Can you work these out from the model? Positions are in its coordinate system, mm. Give positions to 0.01 mm unless a question says otherwise; leave off trailing zeros. Loops run counter-clockwise (first coordinate to the right, second up) from the corner with the lowest first, then second, coordinate; pieces in that order, holes last. Notation, with made-up numbers: (0.25, 19) -> (58.25, 19) arc R33 cw to (58.25, 53) -> close; hole circle Ø11 at (-23.75, -39). An arc over 180 degrees is marked (long way). Return JSON: item names as keys, results as strings. Group by question number.
Q1. I need wall thicknesses on line 1 along Z through (x, y) = (-13, 17.5); line 2 along Y through (x, z) = (27, 0.2); line 3 along X through (y, z) = (-4, 1). Which ranges of each line are inside material? Lowest first, please. Write a range as [from, to].
Q2. Suppose I cut it at A-A, the plane x = 21.5. Please give me the cut outline in (y, z).
Q3. Will this pin go through, and if not, where does the flat tip stop? pin 1 (0.8 mm diameter, centred on y = -9.5, z = 0.5, fed in from -X).
Q4. Suppose I cut it at B-B, the plane y = 16. Please give me the cut outline in (x, z), and give its area (3 significant figures).
```python
from build123d import *

# Parameters (mm, degrees)
F2_W     = 21.7
F2_H     = 24
F3_DEPTH = 2
F4_DEPTH = 1.5
F5_W     = 21.7
F5_H     = 24
F6_DEPTH = 2


with BuildPart() as f3:
    # F2 (on Top) → F3 (new body)
    with BuildSketch(Plane.XY):
        Polygon((32.5, 26.99), (-32.5, 26.99), (-32.5, 24.9966666667), (-10.8, 24.9966666667), (-10.8, 0.9966666667), (-32.5, 0.9966666667), (-32.5, -0.9966666667), (-10.8, -0.9966666667), (-10.8, -24.9966666667), (-32.5, -24.9966666667), (-32.5, -26.99), (32.5, -26.99), (32.5, -24.9966666667), (10.8, -24.9966666667), (10.8, -0.9966666667), (32.5, -0.9966666667), (32.5, 0.9966666667), (10.8, 0.9966666667), (10.8, 24.9966666667), (32.5, 24.9966666667), align=None)
        with Locations((21.65, 12.9966666667)):
            Rectangle(F2_W, F2_H)
        with Locations((-21.65, -12.9966666667)):
            Rectangle(F2_W, F2_H)
        with Locations((-21.65, 12.9966666667)):
            Rectangle(F2_W, F2_H)
        with Locations((21.65, -12.9966666667)):
            Rectangle(F2_W, F2_H)
    extrude(amount=-F3_DEPTH)

    # F2 (on Top) → F4 (join)
    with BuildSketch(Plane.XY):
        Polygon((32.5, 26.99), (-32.5, 26.99), (-32.5, 24.9966666667), (-10.8, 24.9966666667), (-10.8, 0.9966666667), (-32.5, 0.9966666667), (-32.5, -0.9966666667), (-10.8, -0.9966666667), (-10.8, -24.9966666667), (-32.5, -24.9966666667), (-32.5, -26.99), (32.5, -26.99), (32.5, -24.9966666667), (10.8, -24.9966666667), (10.8, -0.9966666667), (32.5, -0.9966666667), (32.5, 0.9966666667), (10.8, 0.9966666667), (10.8, 24.9966666667), (32.5, 24.9966666667), align=None)
    extrude(amount=F4_DEPTH)

    # F5 (on face) → F6 (join)
    with BuildSketch(Plane.XY.offset(1.5)):
        Polygon((10.8, -24.9966666667), (10.8, -0.9966666667), (32.5, -0.9966666667), (32.5, 0.9966666667), (10.8, 0.9966666667), (10.8, 24.9966666667), (32.5, 24.9966666667), (32.5, 26.99), (-32.5, 26.99), (-32.5, 24.9966666667), (-10.8, 24.9966666667), (-10.8, 0.9966666667), (-32.5, 0.9966666667), (-32.5, -0.9966666667), (-10.8, -0.9966666667), (-10.8, -24.9966666667), (-32.5, -24.9966666667), (-32.5, -26.99), (32.5, -26.99), (32.5, -24.9966666667), align=None)
        with Locations((-21.65, 12.9966666667)):
            Rectangle(F5_W, F5_H)
        with Locations((-21.65, -12.9966666667)):
            Rectangle(F5_W, F5_H)
        with Locations((21.65, 12.9966666667)):
            Rectangle(F5_W, F5_H)
        with Locations((21.65, -12.9966666667)):
            Rectangle(F5_W, F5_H)
    extrude(amount=F6_DEPTH)


solid = f3.part
```
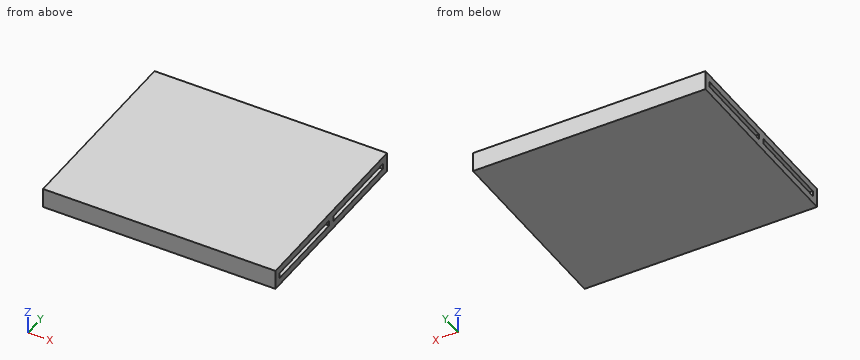
Ans:
{
 "1": {"line 1": "z = [-2, 0], [1.5, 3.5]", "line 2": "y = [-26.99, -25], [-1, 1], [25, 26.99]", "line 3": "x = [-10.8, 10.8]"},
 "2": {"outline": "(-26.99, -2) -> (26.99, -2) -> (26.99, 3.5) -> (-26.99, 3.5) -> close; hole (-25, 0) -> (-1, 0) -> (-1, 1.5) -> (-25, 1.5) -> close; hole (1, 0) -> (25, 0) -> (25, 1.5) -> (1, 1.5) -> close"},
 "3": {"pin 1": "stops at x = -10.8"},
 "4": {"outline": "(-32.5, -2) -> (32.5, -2) -> (32.5, 0) -> (10.8, 0) -> (10.8, 1.5) -> (32.5, 1.5) -> (32.5, 3.5) -> (-32.5, 3.5) -> (-32.5, 1.5) -> (-10.8, 1.5) -> (-10.8, 0) -> (-32.5, 0) -> close", "area": "292 mm^2"}
}
